Here's the drawing with two shaded views (mm, measured from the low corner). I have some questions. A direction names the side the tool comes from. Coordinates: 2 decimals unless noted, no trailing zeros. Loops run counter-clockwise (first coordinate to the right, second up) from the corner with the lowest first, then second, coordinate; pieces in that order, holes last. Notation, with made-up numbers: M -3.75,-28.5 L 6.25,-28.5 A16 ccw 6.25,2.5 Z; hole C 45,-10 d9. An arc over 180 degrees is marked long. Return JSON: item names as keys, results as strings. Group by question number.
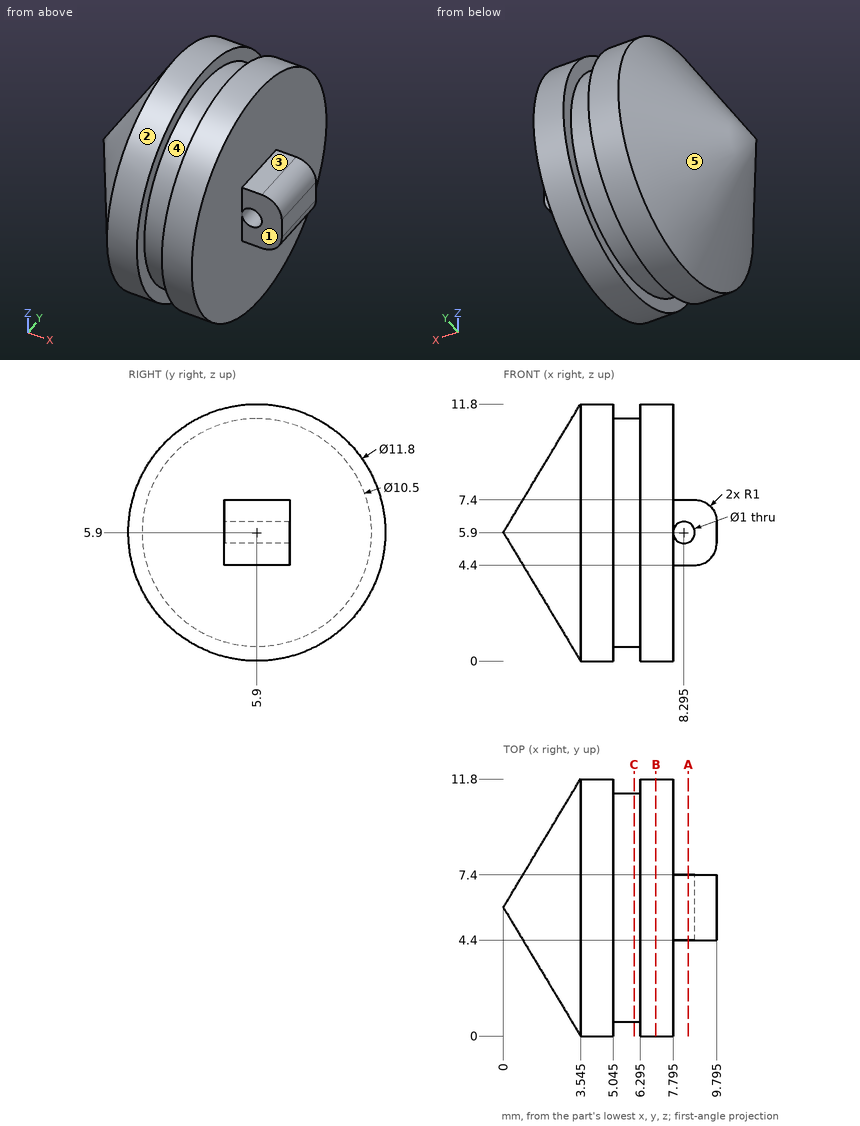
1) Suppose I cut it at B-B, the plane x = 7. List the corners of the cut face in (y, z) for me, then the cut area to 3 significant figures.
2) If I drill on line 1 (Y direction, x = 8, z = 7); line 2 (X direction, y = 5.75, z = 5.9) (3 decimals); line 3 (Y direction, x = 6, z = 6), over which ranges is the centre line in solid material (lowest first)? Write a range as from..to.
3) For pin 1 (0.5 mm diameter, centred on x = 8.5, y = 5.5, fed in from -Z); pin 2 (0.6 mm diameter, centred on x = 9, z = 5.5, fed in from +Y); pin 3 (1.5 mm diameter, centred on x = 4, y = 10.5, fed in from +Z); pin 4 (6 mm diameter, centred on y = 3, z = 4, fed in from +X) (3 decimals), each with a flat end and sliding along its axis, tell me the tip position at first contact or that it passes through.
4) Suppose I cut it at C-C, the plane x = 6. List the corners of the cut face in (y, z) for me, then the cut area to 3 significant figures.
5) For the marked faces 1, 2, 3, 4 and 5, which set-ups out of +Z, -Z, +X, -X, +Y, -Y let a thin tool reach every point of the face, with its end or its side?
6) Suppose I cut it at A-A, the plane x = 8.5. List the corners of the cut face in (y, z) for me.
Returned:
{
 "1": {"outline": "C 5.9,5.9 d11.8", "area": "109 mm²"},
 "2": {"line 1": "y = 4.4..7.4", "line 2": "x = 0.09..7.795, 8.795..9.795", "line 3": "y = 0.65..11.15"},
 "3": {"pin 1": "stops at z = 4.4", "pin 2": "stops at y = 7.4", "pin 3": "stops at z = 10.37", "pin 4": "stops at x = 9.795"},
 "4": {"outline": "C 5.9,5.9 d10.5", "area": "86.6 mm²"},
 "5": {"face 1": "+Z, -Z, +X, -Y", "face 2": "+X, -X", "face 3": "+Z, +X, +Y, -Y", "face 4": "none", "face 5": "-X"},
 "6": {"outline": "M 4.4,4.4 L 7.4,4.4 L 7.4,5.44 L 4.4,5.44 Z; M 4.4,6.36 L 7.4,6.36 L 7.4,7.4 L 4.4,7.4 Z"}
}
